Geometry: final body of the model. Coordinates: model frame, mm. Give positions to 0.01 mm unless a question says otherwise; leave off trailing zeros. Loops run counter-clockwise (first coordinate to the right, second up) from the corner with the lowest first, then second, coordinate; pieces in that order, holes last. Notation, with made-up numbers: (-39, 12.25) - (-18, 12.25) arc R25 ccw to (-18, 29.25) - close; hole circle Ø4 at (9.5, 3.25). An arc over 180 degrees is marked (long way). Use one line per item in the form item = value.
```python
from build123d import *

# Parameters (mm, degrees)
SKETCH_1_R          = 50
EXTRUDE_1_DEPTH     = 29
SKETCH_2_R          = 5
CUT_EXTRUDE_1_DEPTH = 77.426435217
FILLET_1_R          = 5


with BuildPart() as part:
    # 草图1 → 凸台-拉伸1 (new body)
    with BuildSketch(Plane.XY):
        with Locations(Location((0, 0, 0), (0, 0, 180))):
            Circle(SKETCH_1_R)
    extrude(amount=EXTRUDE_1_DEPTH)

    # 草图2 → 切除-拉伸1 (cut, through all)
    with BuildSketch(Plane.XY.offset(29)):
        Circle(SKETCH_2_R)
    extrude(amount=-CUT_EXTRUDE_1_DEPTH, mode=Mode.SUBTRACT)

    # 圆角1
    fillet_1_edges = [part.edges().sort_by_distance(p)[0] for p in [
        (50, 0, 0),
        (50, 0, 29),
    ]]
    fillet(fillet_1_edges, radius=FILLET_1_R)


solid = part.part
```
(1) Pull-direction query (Y, two-part tool) for faces 1 (the face through (-47.69, -15.02, 14.37)), 2 (the face through (1, 9, 0)), 3 (the face through (-1.08, -4.88, 14.7)); classes: released by +Y, released by -Y, zero draft, split by the parting line, or undercut.
Solution:
face_1 = split by the parting line
face_2 = zero draft
face_3 = undercut
(2) Cut plane A-A (x = 0). Return the cut outline in (y, z).
Solution:
outline = (-50, 5) arc R5 ccw to (-45, 0) - (-5, 0) - (-5, 29) - (-45, 29) arc R5 ccw to (-50, 24) - close; (5, 0) - (45, 0) arc R5 ccw to (50, 5) - (50, 24) arc R5 ccw to (45, 29) - (5, 29) - close
(3) Pin query (flat end, axial travel): P1, Ø3, axis at y = -9.5, z = 17.5, coming from the +X side; P2, Ø6, axis at y = -22.5, z = 9, coming from the -X side; P3, Ø10, axis at x = 36.5, z = 16.5, coming from the +Y side. Return the tip coordinate at first contact, or that it passes through.
Solution:
P1 = 49.36
P2 = -46.04
P3 = 38.83
(4) Material intervals for L1, parallel to Y at x = 0, z = 12.75; L2, parallel to Y at x = 1.5, z = 4.75; L3, parallel to X at y = 34, z = 19.25, sorted ascending. Write a range as from..to.
Solution:
L1 = -50..-5, 5..50
L2 = -49.97..-4.77, 4.77..49.97
L3 = -36.66..36.66
(5) Cut plane C-C (z = 22.25). Return the cut outline in (x, y), plus the area to 3 significant figures.
Solution:
outline = circle Ø100 at (0, 0); hole circle Ø10 at (0, 0)
area = 7,780 mm2
